The listing builds one solid part. Answer for the finished solid, in the listing's coordinates (mm). A direction names the side the tool comes from. Give positions to 0.01 mm unless a question says otherwise; leave off trailing zeros. Write each loop counter-clockwise with the first axis right and the second up, starting at its lowest first coordinate (ties: lowest second). Pieces come first, ordered by that corner, then holes.
```python
from build123d import *

# Parameters (mm, degrees)
BASESKETCH_W          = 220
BASESKETCH_H          = 40
BASE_DEPTH            = 3
HOLESSKETCH_R         = 2
HOLES_DEPTH           = 112.843640856
SUPPORTSKETCH_W       = 11
SUPPORTSKETCH_H       = 25
SUPPORTSKETCH_R       = 2
SUPPORTSKETCH_W_2     = 196
SUPPORTSKETCH_H_2     = 40
SUPPORTSKETCH_W_3     = 93.5
SUPPORTSKETCH_H_3     = 15.5
SUPPORT_DEPTH         = 6
CONNECTORSKETCH_W     = 10
CONNECTORSKETCH_H     = 3
CONNECTOR_DEPTH       = 3
WEIGHTREDUCTION_DEPTH = 113.165056947


with BuildPart() as part:
    # BaseSketch → Base (new body)
    with BuildSketch(Plane(origin=(0, 0, 0), x_dir=(1, 0, 0), z_dir=(0, 1, 0))):
        Rectangle(BASESKETCH_W, BASESKETCH_H)
    extrude(amount=BASE_DEPTH)

    # HolesSketch → Holes (cut, through all)
    with BuildSketch(Plane.XZ):
        with Locations(Location((-102.5, 0, 0), (0, 0, 270))):
            Circle(HOLESSKETCH_R)
        with Locations(Location((-80, 0, 0), (0, 0, 270))):
            Circle(HOLESSKETCH_R)
        with Locations(Location((-67.5, 16, 0), (0, 0, 270))):
            Circle(HOLESSKETCH_R)
        with Locations(Location((-67.5, -16, 0), (0, 0, 270))):
            Circle(HOLESSKETCH_R)
        with Locations(Location((102.5, -16, 0), (0, 0, 270))):
            Circle(HOLESSKETCH_R)
        with Locations(Location((102.5, 16, 0), (0, 0, 270))):
            Circle(HOLESSKETCH_R)
    extrude(amount=-HOLES_DEPTH, mode=Mode.SUBTRACT)

    # SupportSketch → Support (add)
    with BuildSketch(Plane(origin=(0, 3, 0), x_dir=(1, 0, 0), z_dir=(0, 1, 0))):
        with Locations((-102.5, 0)):
            Rectangle(SUPPORTSKETCH_W, SUPPORTSKETCH_H)
        with Locations(Location((-102.5, 0, 0), (0, 0, 90))):
            Circle(SUPPORTSKETCH_R, mode=Mode.SUBTRACT)
        with Locations((12, 0)):
            Rectangle(SUPPORTSKETCH_W_2, SUPPORTSKETCH_H_2)
        with Locations(Location((-67.5, -16, 0), (0, 0, 90))):
            Circle(SUPPORTSKETCH_R, mode=Mode.SUBTRACT)
        Polygon((-1.5, -1.5), (-1.5, -17), (-58, -17), (-74, -1.5), align=None, mode=Mode.SUBTRACT)
        with Locations(Location((102.5, -16, 0), (0, 0, 90))):
            Circle(SUPPORTSKETCH_R, mode=Mode.SUBTRACT)
        with Locations((48.25, -9.25)):
            Rectangle(SUPPORTSKETCH_W_3, SUPPORTSKETCH_H_3, mode=Mode.SUBTRACT)
        with Locations(Location((-80, 0, 0), (0, 0, 90))):
            Circle(SUPPORTSKETCH_R, mode=Mode.SUBTRACT)
        Polygon((-58, 17), (-1.5, 17), (-1.5, 1.5), (-74, 1.5), align=None, mode=Mode.SUBTRACT)
        with Locations(Location((-67.5, 16, 0), (0, 0, 90))):
            Circle(SUPPORTSKETCH_R, mode=Mode.SUBTRACT)
        with Locations((48.25, 9.25)):
            Rectangle(SUPPORTSKETCH_W_3, SUPPORTSKETCH_H_3, mode=Mode.SUBTRACT)
        with Locations(Location((102.5, 16, 0), (0, 0, 90))):
            Circle(SUPPORTSKETCH_R, mode=Mode.SUBTRACT)
    extrude(amount=SUPPORT_DEPTH)

    # ConnectorSketch → Connector (add)
    with BuildSketch(Plane(origin=(0, 9, 0), x_dir=(1, 0, 0), z_dir=(0, 1, 0))):
        with Locations((0, -18.5)):
            Rectangle(CONNECTORSKETCH_W, CONNECTORSKETCH_H)
        with Locations((0, 18.5)):
            Rectangle(CONNECTORSKETCH_W, CONNECTORSKETCH_H)
    extrude(amount=CONNECTOR_DEPTH)

    # WeightReductionSketch → WeightReduction (cut, symmetric)
    with BuildSketch(Plane(origin=(0, 9, 0), x_dir=(1, 0, 0), z_dir=(0, 1, 0))):
        Polygon((-74, 1.5), (-58, 17), (-41.949280136, 1.5), align=None)
        Polygon((-55, 17), (-38.949280136, 1.5), (-22.898560272, 17), align=None)
        Polygon((-19.898560272, 17), (-35.949280136, 1.5), (-3.847840409, 1.5), align=None)
        Polygon((-16.898560272, 17), (-1.5, 2.129783197), (-1.5, 17), align=None)
        Polygon((1.5, 2.129783197), (16.898560272, 17), (1.5, 17), align=None)
        Polygon((3.847840409, 1.5), (19.898560272, 17), (35.949280136, 1.5), align=None)
        Polygon((38.949280136, 1.5), (22.898560272, 17), (55, 17), align=None)
        Polygon((41.949280136, 1.5), (58, 17), (74.050719864, 1.5), align=None)
        Polygon((77.050719864, 1.5), (61, 17), (93.101439728, 17), align=None)
        Polygon((95, 15.936352019), (80.050719864, 1.5), (95, 1.5), align=None)
    weightreduction = extrude(amount=WEIGHTREDUCTION_DEPTH, both=True, mode=Mode.SUBTRACT)

    # WeightReductionMirror: WeightReduction across plane
    add(weightreduction.mirror(Plane.XY), mode=Mode.SUBTRACT)


solid = part.part
```
Item 1: Consider probe 1 along Z at (x, y) = (45, 5.5); probe 2 along Z at (x, y) = (102.5, 4); probe 3 along X at (y, z) = (5.75, 0). Determine where each line is inside the solid, lowest interval first.
Conclusion:
probe 1: z = -20 to -17, -1.5 to 1.5, 17 to 20
probe 2: z = -20 to -18, -14 to 14, 18 to 20
probe 3: x = -108 to -104.5, -100.5 to -97, -86 to -82, -78 to 110
Item 2: A cutting plane is placed at A-A, the plane x = -102.5. Give the vertices of the cut face in (y, z), plus the area to 3 significant figures.
Conclusion:
outline: (0, -20) - (3, -20) - (3, -12.5) - (9, -12.5) - (9, -2) - (0, -2) - close; (0, 2) - (9, 2) - (9, 12.5) - (3, 12.5) - (3, 20) - (0, 20) - close
area: 234 mm2
Item 3: A cutting plane is placed at B-B, the plane x = 83. Give the vertices of the cut face in (y, z).
Conclusion:
outline: (0, -20) - (9, -20) - (9, -17) - (0, -17) - close; (0, -7.25) - (3, -7.25) - (3, -4.35) - (0, -4.35) - close; (0, -1.5) - (9, -1.5) - (9, 1.5) - (0, 1.5) - close; (0, 4.35) - (3, 4.35) - (3, 7.25) - (0, 7.25) - close; (0, 17) - (9, 17) - (9, 20) - (0, 20) - close
Item 4: A cutting plane is placed at C-C, the plane z = -9.5. Count the separate pieces of the cut face and the enclosed holes in it, plus the area to 3 significant figures.
Conclusion:
separate pieces: 11
enclosed holes: 0
area: 554 mm2
Item 5: Each of these flat-tipped pins is pushed along its axis until it touches: P1, Ø17, axis at x = 9.5, z = -5.5, coming from the +Y side; P2, Ø4.5, axis at x = -29.5, z = -8, coming from the +Y side; P3, Ø1.8, axis at x = -101, y = 5.5, coming from the +Z side. Where does it stop, or does it pass through?
Conclusion:
P1: stops at y = 9
P2: stops at y = 3
P3: stops at z = 12.5
Item 6: Which of the six approach directions +Z, -Z, +X, -X, +Y, -Y give full straight-line access (tool end or side, diameter ignored) to faces 1 (the face through (-11.76, 1.48, -9.14)), 2 (the face through (67, 3, -9))?
Conclusion:
face 1: +Y, -Y
face 2: +Y
Item 7: A cutting plane is placed at D-D, the plane x = -67.5. Give the vertices of the cut face in (y, z), plus the area to 3 significant figures.
Conclusion:
outline: (0, -20) - (9, -20) - (9, -18) - (0, -18) - close; (0, -14) - (9, -14) - (9, -7.8) - (0, -7.8) - close; (0, -1.5) - (9, -1.5) - (9, 1.5) - (0, 1.5) - close; (0, 7.8) - (9, 7.8) - (9, 14) - (0, 14) - close; (0, 18) - (9, 18) - (9, 20) - (0, 20) - close
area: 175 mm2
Item 8: Determine the mould class of faces 3 (the face through (10, 3, -9)), 4 (the face through (-103, 6, -12.5)), 5 (the face through (-86, 6, 0)) for opening direction Z: pulls with the +Z half, pulls with the -Z half, needs draft (parallel to the pull), parting line crosses it, or undercut.
Conclusion:
face 3: undercut
face 4: pulls with the -Z half
face 5: needs draft
